For this review, take the finished solid that the model builds, in its own axes (mm). A direction names the side the tool comes from. Round coordinates to 2 decimals unless told otherwise and drop trailing zeros. Write each loop counter-clockwise with the first axis right and the second up, starting at its lowest first coordinate (ties: lowest second). Pieces come first, ordered by that corner, then holes. Notation, with made-up numbers: M 75.25,-15 L 85.25,-15 A24 cw 85.25,21 Z; hole C -32.5,25 d11. An arc over 180 degrees is marked long. One line per question, with ' | ' between items.
```python
from build123d import *

# Parameters (mm, degrees)
CROQUIS1_W              = 180
CROQUIS1_H              = 180
SALIENTE_EXTRUIR1_DEPTH = 30.7
CROQUIS2_W              = 180
CROQUIS2_H              = 162.21
CORTAR_EXTRUIR1_DEPTH   = 20.7
CROQUIS3_W              = 10.7
CROQUIS3_H              = 12.79
CORTAR_EXTRUIR2_DEPTH   = 274.7
SALIENTE_EXTRUIR2_DEPTH = 20
CROQUIS5_W              = 10
CROQUIS5_H              = 17.79
CROQUIS5_W_2            = 6.8
CORTAR_EXTRUIR3_DEPTH   = 30.7
CROQUIS6_W              = 6.8
CROQUIS6_H              = 97.21
CROQUIS6_W_2            = 10
CROQUIS6_W_3            = 93.2
CROQUIS6_H_2            = 38
CORTAR_EXTRUIR4_DEPTH   = 5
CHAFL_N1_SIZE           = 15
CHAFL_N1_SIZE2          = 8.660254038
CROQUIS7_R              = 1.4
CORTAR_EXTRUIR5_DEPTH   = 20
CROQUIS8_R              = 4.4
CROQUIS8_R_2            = 1.4
SALIENTE_EXTRUIR3_DEPTH = 3


with BuildPart() as part:
    # Croquis1 → Saliente-Extruir1 (new body)
    with BuildSketch(Plane.XY):
        with Locations((90, 90)):
            Rectangle(CROQUIS1_W, CROQUIS1_H)
    extrude(amount=SALIENTE_EXTRUIR1_DEPTH)

    # Croquis2 → Cortar-Extruir1 (cut)
    with BuildSketch(Plane(origin=(0, 0, 0), x_dir=(-1, 0, 0), z_dir=(0, 0, -1))):
        with Locations((-90, 81.105)):
            Rectangle(CROQUIS2_W, CROQUIS2_H)
    extrude(amount=-CORTAR_EXTRUIR1_DEPTH, mode=Mode.SUBTRACT)

    # Croquis3 → Cortar-Extruir2 (cut)
    with BuildSketch(Plane.ZY):
        with Locations((15.35, 168.605)):
            Rectangle(CROQUIS3_W, CROQUIS3_H)
    extrude(amount=-CORTAR_EXTRUIR2_DEPTH, mode=Mode.SUBTRACT)

    # Croquis4 → Saliente-Extruir2 (add)
    with BuildSketch(Plane(origin=(180, 0, 0), x_dir=(0, 0, -1), z_dir=(1, 0, 0))):
        Polygon((-20.7, 0), (-20.7, 175), (-10, 175), (-10, 162.21), (0, 162.21), (0, 180), (-30.7, 180), (-30.7, 0), align=None)
    extrude(amount=SALIENTE_EXTRUIR2_DEPTH)

    # Croquis5 → Cortar-Extruir3 (cut)
    with BuildSketch(Plane.XY.offset(30.7)):
        Polygon((0, 0), (6.8, 0), (51.8, 0), (51.8, 38), (6.8, 38), (6.8, 65), (0, 65), align=None)
        Polygon((200, 0), (190, 0), (145, 0), (145, 38), (190, 38), (190, 65), (200, 65), align=None)
        with Locations((195, 171.105)):
            Rectangle(CROQUIS5_W, CROQUIS5_H)
        with Locations((3.4, 171.105)):
            Rectangle(CROQUIS5_W_2, CROQUIS5_H)
    extrude(amount=-CORTAR_EXTRUIR3_DEPTH, mode=Mode.SUBTRACT)

    # Croquis6 → Cortar-Extruir4 (cut)
    with BuildSketch(Plane.XY.offset(30.7)):
        with Locations((3.4, 113.605)):
            Rectangle(CROQUIS6_W, CROQUIS6_H)
        with Locations((195, 113.605)):
            Rectangle(CROQUIS6_W_2, CROQUIS6_H)
        with Locations((98.4, 19)):
            Rectangle(CROQUIS6_W_3, CROQUIS6_H_2)
    extrude(amount=-CORTAR_EXTRUIR4_DEPTH, mode=Mode.SUBTRACT)

    # Chaflán1
    chafl_n1_edges = [part.edges().sort_by_distance(p)[0] for p in [
        (98.4, 162.21, 0),
    ]]
    chafl_n1_side = [part.faces().sort_by_distance(p)[0] for p in [
        (98.4, 171.105, 0),
    ]]
    chamfer(chafl_n1_edges, length=CHAFL_N1_SIZE, length2=CHAFL_N1_SIZE2, reference=chafl_n1_side[0])

    # Croquis7 → Cortar-Extruir5 (cut)
    with BuildSketch(Plane.XY.offset(30.7)):
        with Locations((125, 19)):
            Circle(CROQUIS7_R)
        with Locations((71.8, 19)):
            Circle(CROQUIS7_R)
        with Locations((195, 85)):
            Circle(CROQUIS7_R)
        with Locations((195, 142.21)):
            Circle(CROQUIS7_R)
        with Locations(Location((3.4, 142.21, 0), (0, 0, 180))):
            Circle(CROQUIS7_R)
        with Locations(Location((3.4, 85, 0), (0, 0, 180))):
            Circle(CROQUIS7_R)
    extrude(amount=-CORTAR_EXTRUIR5_DEPTH, mode=Mode.SUBTRACT)

    # Croquis8 → Saliente-Extruir3 (add)
    # profile 1 of 2: a face of its own
    with BuildSketch(Plane.XY.offset(30.7)):
        with Locations(Location((56.17, 57.07, 0), (0, 0, 180))):
            Circle(CROQUIS8_R)
        with Locations((56.17, 57.07)):
            Circle(CROQUIS8_R_2, mode=Mode.SUBTRACT)
    # profile 2 of 2: a face of its own
    with BuildSketch(Plane.XY.offset(30.7)):
        with Locations(Location((141.93, 57.07, 0), (0, 0, 180))):
            Circle(CROQUIS8_R)
        with Locations((141.93, 57.07)):
            Circle(CROQUIS8_R_2, mode=Mode.SUBTRACT)
    extrude(amount=SALIENTE_EXTRUIR3_DEPTH)


solid = part.part
```
Item 1: Insertion check: pin 1 Ø3.5 at (x, y) = (3.5, 95.5) entering from +Z; pin 2 Ø4 at (x, z) = (137.5, 5) entering from -Y; pin 3 Ø1.5 at (x, z) = (196, 22.5) entering from -Y. Each pin has a flat end and moves straight along its axis. Give the tip position at first contact, or say it passes through.
Results:
pin 1: z = 25.7 | pin 2: y = 165.09 | pin 3: y = 65
Item 2: Machinability: for faces 1 (the face through (145, 19, 23)), 2 (the face through (99, 86, 20.7)), 3 (the face through (3, 162.21, 23)), 4 (the face through (195, 114, 25.7)), 5 (the face through (3, 114, 25.7)), which of the approach directions +Z, -Z, +X, -X, +Y, -Y give a long, thin tool a straight path to every point of the face, cutting with its end or side? Answer none if there is none.
Results:
face 1: +Z, -Z, +X, -Y | face 2: +X, -X, -Y | face 3: +Z, -Z, -X, +Y | face 4: +Z, +X, +Y, -Y | face 5: +Z, -X, +Y, -Y
Item 3: Take a section at B-B (z = 16). Write out the cut boundary in (x, y).
Results:
outline: M 6.8,175 L 190,175 L 190,180 L 6.8,180 Z
Item 4: Take a section at C-C (z = 28). Write out the cut boundary in (x, y), then the cut area to 3 significant figures.
Results:
outline: M 6.8,38 L 190,38 L 190,180 L 6.8,180 Z | area: 26,000 mm2
Item 5: To check wall thickness, follow line 1 along X through (y, z) = (57, 31); line 2 along X through (y, z) = (142, 23); line 3 along Y through (x, z) = (71.8, 22.3). State the ranges of each line that lie inside material, in increasing order. Write a range as from..to.
Results:
line 1: 51.77..54.77, 57.57..60.57, 137.53..140.53, 143.33..146.33 | line 2: 0..2.02, 4.78..193.62, 196.38..200 | line 3: 0..17.6, 20.4..180
Item 6: Take a section at A-A (x = 150.5). Write out the cut boundary in (y, z), then the cut area to 3 significant figures.
Results:
outline: M 38,20.7 L 175,20.7 L 175,10 L 162.21,10 L 162.21,8.66 L 177.21,0 L 180,0 L 180,30.7 L 38,30.7 Z | area: 1,590 mm2
Item 7: Mouldability with a two-part tool opening along Z and no side actions: class faces 6 (the face through (98, 19, 25.7)), 7 (the face through (100, 38, 27)), 8 (the face through (97, 175, 15)) as +Z half, -Z half, draft (parallel to the pull), parting line (faces both ways), or undercut.
Results:
face 6: +Z half | face 7: draft | face 8: undercut
